Input: part model. Units: mm. Frame: model coordinates. A direction names the side the tool comes from. Coordinates: 2 decimals unless noted, no trailing zeros. Write each loop counter-clockwise with the first axis right and the second up, starting at its lowest first coordinate (ties: lowest second). Pieces come first, ordered by that corner, then holes. Notation, with made-up numbers: M 41.5,8.5 L 64.5,8.5 A29 cw 64.5,42.5 Z; hole C 84.5,-9.5 d5. An arc over 180 degrees is marked long. Write each question's results on one line, items separated by ' | '. Start each with the question number.
1. Ray query, probe 1 along Z at (x, y) = (0.3, 28.5) (3 decimals); probe 2 along Z at (x, y) = (1, 10.5); probe 3 along Z at (x, y) = (-0.25, 17) (3 decimals). Return the intervals inside material, ascending.
2. Set-up query: faces 4 (the flat face through (0, 30, 3.955)), 5 (the flat face through (0, 0, 0)). Return all of +Z, -Z, +X, -X, +Y, -Y with unobstructed straight access to the full face (end or side cutting, diameter ignored); none if empty.
3. Section query C-C, the plane y = 28. Output: boundary loops of the cut face in (x, z) (1 decimal).
4. Section query A-A, the plane x = -1.5. Count the separate pieces of the cut face and the enclosed holes in it, and give its area (3 significant figures).
5. Section query B-B, the plane y = 13. Output: boundary loops of the cut face in (x, z) (1 decimal), and give its area (3 significant figures).
6. First-contact query: pin 1 (1.4 mm diameter, centred on x = 1, y = 35.5, fed in from -Z); pin 2 (1.5 mm diameter, centred on x = 0, y = 7, fed in from -Z); pin 3 (1.4 mm diameter, centred on x = -1, y = 25, fed in from +Z). Flat tips, straight axial feed; report the tip coordinate or a pass-through.
7. Pull-direction query (Y, two-part tool) for faces 1 (the flat face through (0, 18, -9.046)), 2 (the flat face through (2.382, 26, 0)), 3 (the cylindrical face through (0.03, 64.4, -3.61)); classes: +Y half, -Y half, draft (parallel to the pull), parting line (faces both ways), or undercut.
8. Section query D-D, the plane z = -19. Output: boundary loops of the cut face in (x, y), and give its area (3 significant figures).
```python
from build123d import *

# Parameters (mm, degrees)
BOSS_EXTRUDE1_DEPTH  = 2.3815
M3_CLEARANCE_HOLE1_D = 3.2


with BuildPart() as part:
    # Sketch1 → Boss-Extrude1 (new body, symmetric)
    with BuildSketch(Plane(origin=(0, 0, 0), x_dir=(0, 0, -1), z_dir=(1, 0, 0))):
        with BuildLine():
            Line((-22.5, 0), (22.5, 0))
            Line((22.5, 0), (22.5, 4.763))
            Line((22.5, 4.763), (4.677891876, 62.879556228))
            ThreePointArc((4.677891876, 62.879556228), (3.593167148, 64.41232965), (1.809725067, 65))
            Line((1.809725067, 65), (-1.809725067, 65))
            ThreePointArc((-1.809725067, 65), (-3.593167148, 64.41232965), (-4.677891876, 62.879556228))
            Line((-4.677891876, 62.879556228), (-22.5, 4.763))
            Line((-22.5, 4.763), (-22.5, 0))
        make_face()
        with BuildLine():
            Line((-3.955008566, 47), (-3.955008566, 12))
            ThreePointArc((-3.955008566, 12), (-5.305008566, 10.65), (-6.655008566, 12))
            Line((-6.655008566, 12), (-6.655008566, 47))
            ThreePointArc((-6.655008566, 47), (-5.305008566, 48.35), (-3.955008566, 47))
        make_face(mode=Mode.SUBTRACT)
        with BuildLine():
            Line((6.655008566, 47), (6.655008566, 12))
            ThreePointArc((6.655008566, 12), (5.305008566, 10.65), (3.955008566, 12))
            Line((3.955008566, 12), (3.955008566, 47))
            ThreePointArc((3.955008566, 47), (5.305008566, 48.35), (6.655008566, 47))
        make_face(mode=Mode.SUBTRACT)
        with BuildLine():
            Line((12.138351874, 25.164576479), (16.522078624, 12.092233924))
            ThreePointArc((16.522078624, 12.092233924), (16.305639712, 10.660437126), (15.016954073, 10))
            Line((15.016954073, 10), (10.633227322, 10))
            ThreePointArc((10.633227322, 10), (9.510695307, 10.464967985), (9.045727322, 11.5875))
            Line((9.045727322, 11.5875), (9.045727322, 24.659842555))
            ThreePointArc((9.045727322, 24.659842555), (10.377521412, 26.226613354), (12.138351874, 25.164576479))
        make_face(mode=Mode.SUBTRACT)
        with BuildLine():
            Line((-9.045727322, 24.659842555), (-9.045727322, 11.5875))
            ThreePointArc((-9.045727322, 11.5875), (-9.510695307, 10.464967985), (-10.633227322, 10))
            Line((-10.633227322, 10), (-15.016954073, 10))
            ThreePointArc((-15.016954073, 10), (-16.305639712, 10.660437126), (-16.522078624, 12.092233924))
            Line((-16.522078624, 12.092233924), (-12.138351874, 25.164576479))
            ThreePointArc((-12.138351874, 25.164576479), (-10.377521412, 26.226613354), (-9.045727322, 24.659842555))
        make_face(mode=Mode.SUBTRACT)
    extrude(amount=BOSS_EXTRUDE1_DEPTH, both=True)

    # M3 Clearance Hole1 (through all)
    with Locations(Plane(origin=(2.3815, 0, 0), x_dir=(0, 0, -1), z_dir=(1, 0, 0))):
        with Locations((-11.25, 2.3815), (11.25, 2.3815)):
            Hole(M3_CLEARANCE_HOLE1_D / 2)


solid = part.part
```
Answer:
1) probe 1: -15.221 to -6.655, -3.955 to 3.955, 6.655 to 15.221 | probe 2: -20.74 to -16.17, -9.48 to 9.48, 16.17 to 20.74 | probe 3: -18.747 to -14.876, -9.046 to -6.655, -3.955 to 3.955, 6.655 to 9.046, 14.876 to 18.747
2) face 4: +X, -X | face 5: +Z, -Z, +X, -X, -Y
3) outline: M -2.4,-15.4 L 2.4,-15.4 L 2.4,-6.7 L -2.4,-6.7 Z; M -2.4,-4 L 2.4,-4 L 2.4,4 L -2.4,4 Z; M -2.4,6.7 L 2.4,6.7 L 2.4,15.4 L -2.4,15.4 Z
4) separate pieces: 1 | enclosed holes: 6 | area: 1,420 mm^2
5) outline: M -2.4,-20 L 2.4,-20 L 2.4,-16.2 L -2.4,-16.2 Z; M -2.4,-9 L 2.4,-9 L 2.4,-6.7 L -2.4,-6.7 Z; M -2.4,-4 L 2.4,-4 L 2.4,4 L -2.4,4 Z; M -2.4,6.7 L 2.4,6.7 L 2.4,9 L -2.4,9 Z; M -2.4,16.2 L 2.4,16.2 L 2.4,20 L -2.4,20 Z | area: 96.2 mm^2
6) pin 1: z = -13.29 | pin 2: z = -22.04 | pin 3: z = 16.51
7) face 1: undercut | face 2: draft | face 3: +Y half
8) outline: M -2.38,0 L 2.38,0 L 2.38,16.18 L -2.38,16.18 Z | area: 77.0 mm^2
